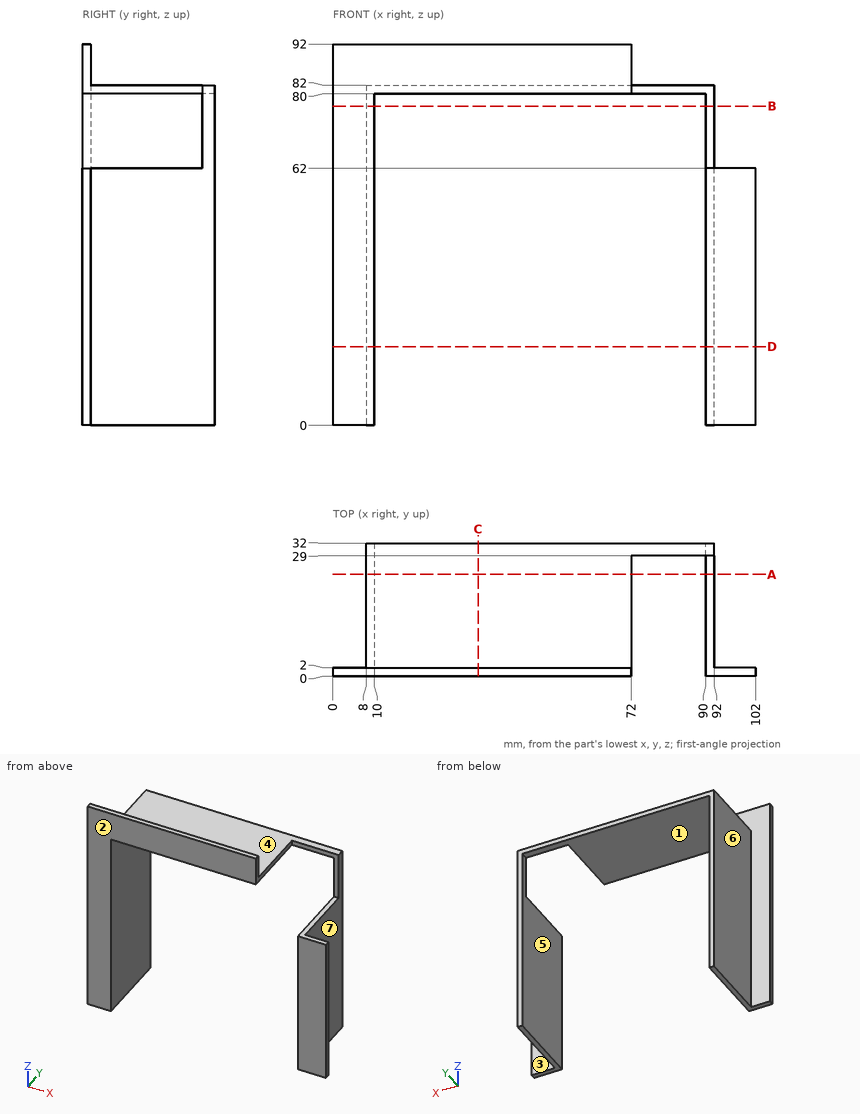
Print and shaded views of the part. All mm, measured from the part's lowest x, y and z. A direction names the side the tool comes from. Coordinates: 2 decimals unless noted, no trailing zeros. Loops run counter-clockwise (first coordinate to the right, second up) from the corner with the lowest first, then second, coordinate; pieces in that order, holes last. Notation, with made-up numbers: (44, -37) - (75, -37) arc R31 ccw to (75, -12) - close; hole circle Ø5 at (43.25, -13). An arc over 180 degrees is marked (long way). Write item = value, one per line. Start each with the question number.
Item 1: Saw through at B-B, the plane z = 77. List the corners of the cut face in (x, y), then the cut area to 3 significant figures.
Item 2: Saw through at D-D, the plane z = 19. List the corners of the cut face in (x, y).
Item 3: Wall check: probe 1 along X at (y, z) = (30, 70.5); probe 2 along Z at (x, y) = (58, 18.5); probe 3 along Y at (x, z) = (7, 52). Give the ranges that are in metal, low to high. Write a range as [from, to].
Item 4: Pull direction X, two halves, no side cores. Call the marked faces 4, 5, 6 and 7: +X half, -X half, draft (parallel to the pull), parting line (faces both ways), or undercut.
Item 5: Drop flat-ended pins along their axis: pin 1 Ø8 at (x, y) = (61, 10) entering from -Z; pin 2 Ø9.5 at (x, y) = (96.5, 8.5) entering from +Z; pin 3 Ø9.5 at (y, z) = (20, 39.5) entering from +X. Give the stop position or say it passes through.
Item 6: 3-axis set-ups, long thin cutter, end or side, ignore diameter. For the marked faces 1, 2 and 3: which of +Z, -Z, +X, -X, +Y, -Y reach the whole face in a straight line?
Item 7: Saw through at C-C, the plane x = 35. List the corners of the cut face in (y, z).
Item 8: Saw through at A-A, the plane y = 24.5. List the corners of the cut face in (x, z).
Answers:
q1.outline = (0, 0) - (10, 0) - (10, 32) - (8, 32) - (8, 2) - (0, 2) - close; (90, 29) - (92, 29) - (92, 32) - (90, 32) - close
q1.area = 86.0 mm2
q2.outline = (0, 0) - (10, 0) - (10, 32) - (8, 32) - (8, 2) - (0, 2) - close; (90, 0) - (102, 0) - (102, 2) - (92, 2) - (92, 32) - (90, 32) - close
q3.probe_1 = [8, 10], [90, 92]
q3.probe_2 = [80, 82]
q3.probe_3 = [0, 2]
q4.face_4 = draft
q4.face_5 = undercut
q4.face_6 = -X half
q4.face_7 = +X half
q5.pin_1 = 80
q5.pin_2 = 62
q5.pin_3 = 92
q6.face_1 = -Z, +Y, -Y
q6.face_2 = +Z, -Z, +X, -X, -Y
q6.face_3 = +Z, -Z, +X, +Y
q7.outline = (0, 80) - (32, 80) - (32, 82) - (2, 82) - (2, 92) - (0, 92) - close
q8.outline = (8, 0) - (10, 0) - (10, 80) - (72, 80) - (72, 82) - (8, 82) - close; (90, 0) - (92, 0) - (92, 62) - (90, 62) - close
